Autodesk Inventor part; units mm, degrees
ref_plane "YZ Plane" through (0, 0, 0) normal (1, 0, 0) x (0, 1, 0)
ref_plane "XZ Plane" through (0, 0, 0) normal (0, 1, 0) x (-1, 0, 0)
ref_plane "XY Plane" through (0, 0, 0) normal (0, 0, 1) x (1, 0, 0)
sketch "Sketch1" plane through (0, 0, 0) normal (0, 0, 1) x (1, 0, 0)
  circle A0 centre (0, 0) radius 27.9
  line L0 (-24, 12.5) -> (24, 12.5)
  line L1 (24, 12.5) -> (24, -12.5)
  line L2 (24, -12.5) -> (-24, -12.5)
  line L3 (-24, -12.5) -> (-24, 12.5)
  dimension "d0" = 55.8
  dimension "d1" = 48
  dimension "d2" = 24
  dimension "d3" = 25
  dimension "d4" = 12.5
extrude "Extrusion1" add sketch "Sketch1" along normal mid plane 15
fillet "Fillet1" radius 1 8 edges at (0, 12.5, 7.5) (-24, 0, 7.5) (0, -12.5, 7.5) (24, 0, 7.5) (0, 12.5, -7.5) (-24, 0, -7.5) (0, -12.5, -7.5) (24, 0, -7.5)
properties part number "soporte central pila"
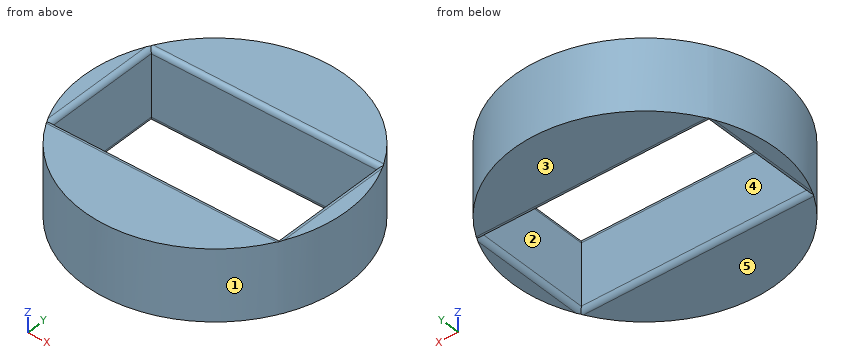
Here's how the part is built. I have some questions about the finished solid (model axes, mm). Face numbers are marked on the shaded views. A direction names the side the tool comes from. Round coordinates to 2 decimals unless told otherwise and drop trailing zeros. Order: outer loops, then holes, each group sorted by start corner. A loop starts at its lowest first (then second) coordinate and runs counter-clockwise, first axis right, second up. Notation, with made-up numbers: (32, 85) -> (58, 85) arc R22 cw to (58, 122) -> close; hole circle Ø6 at (38.5, 73). An arc over 180 degrees is marked (long way). Return JSON: item names as keys, results as strings.
Q1. If we section it at D-D on y = 19.5: List the corners of the cut face in (x, z) for me.
Filled sheet:
{"outline": "(-19.95, -7.5) -> (19.95, -7.5) -> (19.95, 7.5) -> (-19.95, 7.5) -> close"}
Q2. If we mould it in two halves opening along Y, with no side actions, what happens to the marked faces 1, 2 and 3? For each: released by +Y, released by -Y, zero draft, split by the parting line, or undercut.
Filled sheet:
{"face 1": "split by the parting line", "face 2": "undercut", "face 3": "zero draft"}
Q3. If we section it at C-C on z = -1: List the corners of the cut face in (x, y) for me, plus the area to 3 significant figures.
Filled sheet:
{"outline": "circle Ø55.8 at (0, 0); hole (-24, -12.5) -> (24, -12.5) -> (24, 12.5) -> (-24, 12.5) -> close", "area": "1,250 mm^2"}
Q4. If we section it at B-B on x = 0: List the corners of the cut face in (y, z) for me, plus the area to 3 significant figures.
Filled sheet:
{"outline": "(-27.9, -7.5) -> (-13.5, -7.5) arc R1 ccw to (-12.5, -6.5) -> (-12.5, 6.5) arc R1 ccw to (-13.5, 7.5) -> (-27.9, 7.5) -> close; (12.5, -6.5) arc R1 ccw to (13.5, -7.5) -> (27.9, -7.5) -> (27.9, 7.5) -> (13.5, 7.5) arc R1 ccw to (12.5, 6.5) -> close", "area": "461 mm^2"}
Q5. I need wall thicknesses on line 1 along X through (y, z) = (25, 5); line 2 along Y through (x, z) = (13.5, 6); line 3 along Y through (x, z) = (-16.5, -3.25). Which ranges of each line are inside material? Lowest first, please. Write a range as from..to.
Filled sheet:
{"line 1": "x = -12.39..12.39", "line 2": "y = -24.42..-12.5, 12.5..24.42", "line 3": "y = -22.5..-12.5, 12.5..22.5"}
Q6. Which directions (+Z, -Z, +X, -X, +Y, -Y) give clear straight access to the entire face, cutting with the end or side of a thin tool? Please do the marked faces 4 and 5.
Filled sheet:
{"face 4": "+Z, -Z", "face 5": "-Z, +X, -X, +Y, -Y"}
Q7. For pin 1 Ø4 at (y, z) = (-6, -1.5) entering from -X; pin 2 Ø5 at (x, z) = (8, -5) entering from -Y; pin 3 Ø3 at (y, z) = (8, 1.5) entering from +X, each with a flat end and sliding along its axis, tell me the tip position at first contact or that it passes through.
Filled sheet:
{"pin 1": "stops at x = -27.61", "pin 2": "stops at y = -27.35", "pin 3": "stops at x = 27.13"}
Q8. If we section it at A-A on y = 0: List the corners of the cut face in (x, z) for me, plus the area to 3 significant figures.
Filled sheet:
{"outline": "(-27.9, -7.5) -> (-25, -7.5) arc R1 ccw to (-24, -6.5) -> (-24, 6.5) arc R1 ccw to (-25, 7.5) -> (-27.9, 7.5) -> close; (24, -6.5) arc R1 ccw to (25, -7.5) -> (27.9, -7.5) -> (27.9, 7.5) -> (25, 7.5) arc R1 ccw to (24, 6.5) -> close", "area": "116 mm^2"}
